```python
from build123d import *

# Parameters (mm, degrees)
BOSS_EXTRUDE1_DEPTH = 24
SKETCH5_W           = 20
SKETCH5_H           = 30.196049995
CUT_EXTRUDE1_DEPTH  = 20
SKETCH6_R           = 0.625
BOSS_EXTRUDE2_DEPTH = 20


with BuildPart() as part:
    # Sketch2 → Boss-Extrude1 (new body)
    with BuildSketch(Plane(origin=(0, 0, 0), x_dir=(0, 0, -1), z_dir=(1, 0, 0))):
        Polygon((0, 0), (70, 0), (70, 2), (48.984631039, 2), (2, 19.101007166), (2, 41.400415076), (-7.490496191, 44.854673198), (-8.174536478, 42.975287957), (0, 40), align=None)
    extrude(amount=BOSS_EXTRUDE1_DEPTH)

    # Sketch5 → Cut-Extrude1 (cut)
    with BuildSketch(Plane(origin=(0, 0, -2), x_dir=(-1, 0, 0), z_dir=(0, 0, -1))):
        with Locations((-12, 34.199032164)):
            Rectangle(SKETCH5_W, SKETCH5_H)
    extrude(amount=-CUT_EXTRUDE1_DEPTH, mode=Mode.SUBTRACT)

    # Sketch6 → Boss-Extrude2 (add)
    with BuildSketch(Plane(origin=(2, 0, 0), x_dir=(0, 0, -1), z_dir=(1, 0, 0))):
        with Locations(Location((-6.892823714, 43.572960434, 0), (0, 0, 270))):
            Circle(SKETCH6_R)
    extrude(amount=BOSS_EXTRUDE2_DEPTH)


solid = part.part
```
Model file for the job. Use its own axes, mm. A direction names the side the tool comes from. Coordinates: 2 decimals unless noted, no trailing zeros. Loops run counter-clockwise (first coordinate to the right, second up) from the corner with the lowest first, then second, coordinate; pieces in that order, holes last. Notation, with made-up numbers: (-5, 46.5) -> (45, 46.5) arc R22 ccw to (45, 76.5) -> close; hole circle Ø1 at (81, 26.25). An arc over 180 degrees is marked (long way). Answer as a JSON object with one key per item and string values.
Q1. Probe probe 1 along X at (y, z) = (23.5, -1.5); probe 2 along Y at (x, z) = (19.75, -52.5); probe 3 along Y at (x, z) = (15.25, -1.5). List the from-to ranges inside material, lowest first.
Report:
{"probe 1": "x = 0 to 2, 22 to 24", "probe 2": "y = 0 to 2", "probe 3": "y = 0 to 19.1"}
Q2. Cut at A-A (y = 29). List the corners of the cut face in (x, z), and give its area (3 significant figures).
Report:
{"outline": "(0, -2) -> (2, -2) -> (2, 0) -> (0, 0) -> close; (22, -2) -> (24, -2) -> (24, 0) -> (22, 0) -> close", "area": "8.00 mm2"}
Q3. Cut at B-B (x = 4.5). List the corners of the cut face in (y, z) (3 decimals), and give its area (3 significant figures).
Report:
{"outline": "(0, -70) -> (2, -70) -> (2, -48.985) -> (19.101, -2) -> (19.101, 0) -> (0, 0) -> close; circle Ø1.25 at (43.573, 6.893)", "area": "577 mm2"}
Q4. Cut at D-D (y = 8). List the corners of the cut face in (x, z).
Report:
{"outline": "(0, -32.5) -> (24, -32.5) -> (24, 0) -> (0, 0) -> close"}
Q5. Pull direction X, two halves, no side cores. Call faces 5 (the flat face through (24, 9, -19)), 6 (the flat face through (0, 9, -19)), 7 (the flat face through (12, 2, -60)), 8 (the flat face through (22, 34, -1)): released by +X, released by -X, zero draft, split by the parting line, or undercut.
Report:
{"face 5": "released by +X", "face 6": "released by -X", "face 7": "zero draft", "face 8": "undercut"}
Q6. 3-axis set-ups, long thin cutter, end or side, ignore diameter. For faces 1 (the flat face through (12, 19.101, -1)), 2 (the flat face through (22.986, 43.928, 7.828)), 3 (the flat face through (12, 11, 0)), 4 (the flat face through (23, 30, -2)): which of +Z, -Z, +X, -X, +Y, -Y reach the whole face in a straight line?
Report:
{"face 1": "+Z, -Z, +Y", "face 2": "+Z, +X, -X, +Y", "face 3": "+Z, +X, -X, -Y", "face 4": "-Z, +X, -X, +Y"}
Q7. Cut at C-C (z = -64.5). List the corners of the cut face in (x, y), and give its area (3 significant figures).
Report:
{"outline": "(0, 0) -> (24, 0) -> (24, 2) -> (0, 2) -> close", "area": "48.0 mm2"}
Q8. Flat gauge pins, fed straight in: P1, Ø7, axis at x = 13.5, y = 20, coming from the +Z side; P2, Ø0.6, axis at x = 1.5, y = 34.5, coming from the -Z side; P3, Ø5, axis at y = 37, z = 4.5, coming from the -X side; P4, Ø4, axis at x = 10.5, z = -61, coming from the +Y side. Where does each tip first touch, or does it go through?
Report:
{"P1": "stops at z = 0", "P2": "stops at z = -2", "P3": "passes through", "P4": "stops at y = 2"}
